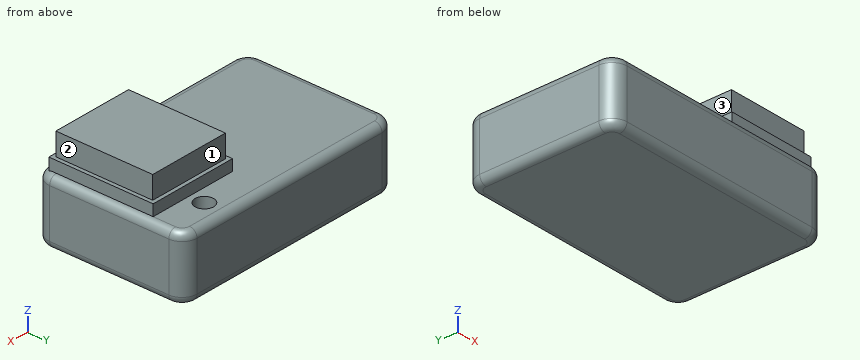
```python
from build123d import *

# Parameters (mm, degrees)
F0_W         = 32
F0_H         = 20
F0_W_2       = 12
F0_H_2       = 14
F0_R         = 1.25
F0_W_3       = 11
F0_H_3       = 13
F1_DEPTH     = 8.5
F2_DEPTH     = 5
F3_R         = 2
F4_DEPTH     = 13
F5_DEPTH     = 10
F6_T1_DEPTH  = 28
F6_T3_DEPTH  = 16
F6_T6_ANGLE  = 90
F6_T8_ANGLE  = 90
F6_T10_ANGLE = 90
F6_T12_ANGLE = 90
F6_T14_ANGLE = 90
F6_T16_ANGLE = 90
F6_T20_ANGLE = 90
F6_T26_ANGLE = 90
F6_T32_ANGLE = 90
F6_T36_ANGLE = 90


# Not quite as in the source:
# - a fillet or chamfer that OpenCascade refuses, or shapes differently, is made with other operations: its cross-section is extruded or revolved along the edge and cut away or added


with BuildPart() as f1:
    # F0 (on Top) → F1 (new body)
    with BuildSketch(Plane.XY):
        Rectangle(F0_W, F0_H)
        with Locations((9, -2)):
            Rectangle(F0_W_2, F0_H_2, mode=Mode.SUBTRACT)
        with Locations((9.5, 7)):
            Circle(F0_R, mode=Mode.SUBTRACT)
        with Locations((9, -2)):
            Rectangle(F0_W_2, F0_H_2)
        with Locations((9, -2)):
            Rectangle(F0_W_3, F0_H_3, mode=Mode.SUBTRACT)
        with Locations((9, -2)):
            Rectangle(F0_W_3, F0_H_3)
    extrude(amount=F1_DEPTH)

    # F0 (on Top) → F2 (join)
    with BuildSketch(Plane.XY):
        with Locations((9.5, 7)):
            Circle(F0_R)
    extrude(amount=F2_DEPTH)

    # F3
    f3_edges = [f1.edges().sort_by_distance(p)[0] for p in [
        (-16, 10, 4.25),
        (-16, -10, 4.25),
        (16, -10, 4.25),
        (16, 10, 4.25),
    ]]
    fillet(f3_edges, radius=F3_R)

    # F0 (on Top) → F4 (join)
    with BuildSketch(Plane.XY):
        with Locations((9, -2)):
            Rectangle(F0_W_3, F0_H_3)
    extrude(amount=F4_DEPTH)

    # F0 (on Top) → F5 (join)
    with BuildSketch(Plane.XY):
        with Locations((9, -2)):
            Rectangle(F0_W_2, F0_H_2)
        with Locations((9, -2)):
            Rectangle(F0_W_3, F0_H_3, mode=Mode.SUBTRACT)
    extrude(amount=F5_DEPTH)

    # F6: fillet of radius 1 on 18 edges, made by hand

    # F6_s2 → F6_t1 (cut)
    with BuildSketch(Plane.YZ.offset(-14)):
        with BuildLine():
            ThreePointArc((-9, 0), (-9.7071067812, 0.2928932188), (-10, 1))
            Line((-10, 1), (-10, 0))
            Line((-10, 0), (-9, 0))
        make_face()
        with BuildLine():
            ThreePointArc((-9, 8.5), (-9.7071067812, 8.2071067812), (-10, 7.5))
            Line((-10, 7.5), (-10, 8.5))
            Line((-10, 8.5), (-9, 8.5))
        make_face()
        with BuildLine():
            ThreePointArc((10, 1), (9.7071067812, 0.2928932188), (9, 0))
            Line((9, 0), (10, 0))
            Line((10, 0), (10, 1))
        make_face()
        with BuildLine():
            ThreePointArc((10, 7.5), (9.7071067812, 8.2071067812), (9, 8.5))
            Line((9, 8.5), (10, 8.5))
            Line((10, 8.5), (10, 7.5))
        make_face()
    extrude(amount=F6_T1_DEPTH, mode=Mode.SUBTRACT)

    # F6_s4 → F6_t3 (cut)
    with BuildSketch(Plane.XZ.offset(-8)):
        with BuildLine():
            ThreePointArc((-15, 0), (-15.7071067812, 0.2928932188), (-16, 1))
            Line((-16, 1), (-16, 0))
            Line((-16, 0), (-15, 0))
        make_face()
        with BuildLine():
            ThreePointArc((15, 0), (15.7071067812, 0.2928932188), (16, 1))
            Line((16, 1), (16, 0))
            Line((16, 0), (15, 0))
        make_face()
        with BuildLine():
            ThreePointArc((15, 8.5), (15.7071067812, 8.2071067812), (16, 7.5))
            Line((16, 7.5), (16, 8.5))
            Line((16, 8.5), (15, 8.5))
        make_face()
        with BuildLine():
            ThreePointArc((-15, 8.5), (-15.7071067812, 8.2071067812), (-16, 7.5))
            Line((-16, 7.5), (-16, 8.5))
            Line((-16, 8.5), (-15, 8.5))
        make_face()
    extrude(amount=F6_T3_DEPTH, mode=Mode.SUBTRACT)

    # F6_s5 → F6_t6 (revolve, cut)
    with BuildSketch(Plane.YZ.offset(-14)):
        with BuildLine():
            ThreePointArc((9, 0), (9.7071067812, 0.2928932188), (10, 1))
            Line((10, 1), (10, 0))
            Line((10, 0), (9, 0))
        make_face()
    revolve(axis=Axis((-14, 8, 0), (0, 0, 1)), revolution_arc=F6_T6_ANGLE, mode=Mode.SUBTRACT)

    # F6_s7 → F6_t8 (revolve, cut)
    with BuildSketch(Plane.XZ.offset(8)):
        with BuildLine():
            ThreePointArc((-15, 0), (-15.7071067812, 0.2928932188), (-16, 1))
            Line((-16, 1), (-16, 0))
            Line((-16, 0), (-15, 0))
        make_face()
    revolve(axis=Axis((-14, -8, 0), (0, 0, 1)), revolution_arc=F6_T8_ANGLE, mode=Mode.SUBTRACT)

    # F6_s9 → F6_t10 (revolve, cut)
    with BuildSketch(Plane.XZ.offset(8)):
        with BuildLine():
            ThreePointArc((15, 0), (15.7071067812, 0.2928932188), (16, 1))
            Line((16, 1), (16, 0))
            Line((16, 0), (15, 0))
        make_face()
    revolve(axis=Axis((14, -8, 0), (0, 0, -1)), revolution_arc=F6_T10_ANGLE, mode=Mode.SUBTRACT)

    # F6_s11 → F6_t12 (revolve, cut)
    with BuildSketch(Plane.YZ.offset(14)):
        with BuildLine():
            ThreePointArc((9, 0), (9.7071067812, 0.2928932188), (10, 1))
            Line((10, 1), (10, 0))
            Line((10, 0), (9, 0))
        make_face()
    revolve(axis=Axis((14, 8, 0), (0, 0, -1)), revolution_arc=F6_T12_ANGLE, mode=Mode.SUBTRACT)

    # F6_s13 → F6_t14 (revolve, cut)
    with BuildSketch(Plane.YZ.offset(14)):
        with BuildLine():
            ThreePointArc((10, 7.5), (9.7071067812, 8.2071067812), (9, 8.5))
            Line((9, 8.5), (10, 8.5))
            Line((10, 8.5), (10, 7.5))
        make_face()
    revolve(axis=Axis((14, 8, 8.5), (0, 0, -1)), revolution_arc=F6_T14_ANGLE, mode=Mode.SUBTRACT)

    # F6_s15 → F6_t16 (revolve, cut)
    with BuildSketch(Plane.YZ.offset(-14)):
        with BuildLine():
            ThreePointArc((10, 7.5), (9.7071067812, 8.2071067812), (9, 8.5))
            Line((9, 8.5), (10, 8.5))
            Line((10, 8.5), (10, 7.5))
        make_face()
    revolve(axis=Axis((-14, 8, 8.5), (0, 0, 1)), revolution_arc=F6_T16_ANGLE, mode=Mode.SUBTRACT)


with BuildPart() as f6_tool18:
    # F6_s19 → F6_t20 (revolve)
    with BuildSketch(Plane.XZ.offset(8)):
        with BuildLine():
            ThreePointArc((15, 8.5), (15.7071067812, 8.2071067812), (16, 7.5))
            Line((16, 7.5), (16, 8.5))
            Line((16, 8.5), (15, 8.5))
        make_face()
    revolve(axis=Axis((14, -8, 8.5), (0, 0, -1)), revolution_arc=F6_T20_ANGLE)

    split(bisect_by=Plane.YZ.offset(15), keep=Keep.TOP)

    split(bisect_by=Plane.XZ.offset(9), keep=Keep.BOTTOM)


with BuildPart() as f1_1:
    add(f1.part)

    # F6_t17: cut F6_tool18
    add(f6_tool18.part, mode=Mode.SUBTRACT)


with BuildPart() as f6_tool24:
    # F6_s25 → F6_t26 (revolve)
    with BuildSketch(Plane.XZ.offset(8)):
        with BuildLine():
            ThreePointArc((15, 8.5), (15.7071067812, 8.2071067812), (16, 7.5))
            Line((16, 7.5), (16, 8.5))
            Line((16, 8.5), (15, 8.5))
        make_face()
    revolve(axis=Axis((14, -8, 8.5), (0, 0, -1)), revolution_arc=F6_T26_ANGLE)

    split(bisect_by=Plane.YZ.offset(15), keep=Keep.BOTTOM)

    split(bisect_by=Plane.XZ.offset(9), keep=Keep.TOP)


with BuildPart() as f1_2:
    add(f1_1.part)

    # F6_t23: cut F6_tool24
    add(f6_tool24.part, mode=Mode.SUBTRACT)


with BuildPart() as f6_tool30:
    # F6_s31 → F6_t32 (revolve)
    with BuildSketch(Plane.XZ.offset(8)):
        with BuildLine():
            ThreePointArc((15, 8.5), (15.7071067812, 8.2071067812), (16, 7.5))
            Line((16, 7.5), (16, 8.5))
            Line((16, 8.5), (15, 8.5))
        make_face()
    revolve(axis=Axis((14, -8, 8.5), (0, 0, -1)), revolution_arc=F6_T32_ANGLE)

    split(bisect_by=Plane.YZ.offset(15), keep=Keep.TOP)

    split(bisect_by=Plane.XZ.offset(9), keep=Keep.TOP)


with BuildPart() as f1_3:
    add(f1_2.part)

    # F6_t29: cut F6_tool30
    add(f6_tool30.part, mode=Mode.SUBTRACT)

    # F6_s35 → F6_t36 (revolve, cut)
    with BuildSketch(Plane.XZ.offset(8)):
        with BuildLine():
            ThreePointArc((-15, 8.5), (-15.7071067812, 8.2071067812), (-16, 7.5))
            Line((-16, 7.5), (-16, 8.5))
            Line((-16, 8.5), (-15, 8.5))
        make_face()
    revolve(axis=Axis((-14, -8, 8.5), (0, 0, 1)), revolution_arc=F6_T36_ANGLE, mode=Mode.SUBTRACT)


solid = f1_3.part
```
The listing builds one solid part. Answer for the finished solid, in the listing's coordinates (mm). Face numbers are marked on the shaded views. A direction names the side the tool comes from. Coordinates: 2 decimals unless noted, no trailing zeros. Write each loop counter-clockwise with the first axis right and the second up, starting at its lowest first coordinate (ties: lowest second). Pieces come first, ordered by that corner, then holes. Notation, with made-up numbers: (-1.75, 19.5) -> (43.25, 19.5) arc R35 cw to (43.25, 54.5) -> close; hole circle Ø6 at (68, 79.25). An arc over 180 degrees is marked (long way). Write each question's results on one line, items separated by ' | '. Start each with the question number.
1) A tool of negligible diameter and unlimited length cuts with its end or side. For the marked faces 1, 2 and 3, from which of +Z, -Z, +X, -X, +Y, -Y can it reach the whole face along a straight path? Write none if from no direction.
2) Straight lines are drawn through the part: probe 1 along Y at (x, z) = (9.5, 6.3); probe 2 along Z at (x, y) = (-5, -5.25); probe 3 along X at (y, z) = (-8, 9.5). For each, find the intervals that lie inside material, in ascending order.
3) Flat-ended cylindrical pins translate along their axes: pin 1 Ø3.5 at (x, z) = (9.5, 12) entering from -Y; pin 2 Ø1.6 at (y, z) = (0.5, 9) entering from -X; pin 3 Ø1.5 at (y, z) = (0, 11.5) entering from +X. Find the tip coordinate at first contact, or state that the pin passes through.
4) A cutting plane is placed at D-D (z = 8). Determine the outline of the cut face in (x, y).
5) A cutting plane is placed at A-A (x = 9.5). Determine the outline of the cut face in (y, z).
6) A cutting plane is placed at B-B (y = 7). Determine the outline of the cut face in (x, z), then the cut area to 3 significant figures.
7) A cutting plane is placed at C-C (z = 12). Determine the outline of the cut face in (x, y).
Values follow:
1) face 1: +Z, +X, -X, +Y | face 2: +Z, +X, +Y, -Y | face 3: +Z, -X, +Y, -Y
2) probe 1: -10 to 5.75, 8.25 to 10 | probe 2: 0 to 8.5 | probe 3: 3 to 15
3) pin 1: y = -8.5 | pin 2: x = -15.71 | pin 3: x = 14.5
4) outline: (-15.87, -8) arc R1.87 ccw to (-14, -9.87) -> (14, -9.87) arc R1.87 ccw to (15.87, -8) -> (15.87, 8) arc R1.87 ccw to (14, 9.87) -> (-14, 9.87) arc R1.87 ccw to (-15.87, 8) -> close; hole circle Ø2.5 at (9.5, 7)
5) outline: (-10, 1) arc R1 ccw to (-9, 0) -> (9, 0) arc R1 ccw to (10, 1) -> (10, 7.5) arc R1 ccw to (9, 8.5) -> (8.25, 8.5) -> (8.25, 5) -> (5.75, 5) -> (5.75, 8.5) -> (5, 8.5) -> (5, 10) -> (4.5, 10) -> (4.5, 13) -> (-8.5, 13) -> (-8.5, 10) -> (-9, 10) -> (-9, 8.5) arc R1 ccw to (-10, 7.5) -> close
6) outline: (-16, 1) arc R1 ccw to (-15, 0) -> (15, 0) arc R1 ccw to (16, 1) -> (16, 7.5) arc R1 ccw to (15, 8.5) -> (10.75, 8.5) -> (10.75, 5) -> (8.25, 5) -> (8.25, 8.5) -> (-15, 8.5) arc R1 ccw to (-16, 7.5) -> close | area: 262 mm²
7) outline: (3.5, -8.5) -> (14.5, -8.5) -> (14.5, 4.5) -> (3.5, 4.5) -> close
